from build123d import *

# Parameters (mm, degrees)
EXTRUDE_1_DEPTH     = 2
FILLET_1_R          = 10
SKETCH_3_R          = 2.1
SKETCH_3_R_2        = 5
CUT_EXTRUDE_1_DEPTH = 3


with BuildPart() as part:
    # 草图1 → 凸台-拉伸1 (new body)
    with BuildSketch(Plane.XY):
        Polygon((75, 117), (-75, 117), (-75, 66.5), (-50, 66.5), (-50, 10), (-75, 10), (-75, -117), (75, -117), (75, 10), (50, 10), (50, 66.5), (75, 66.5), align=None)
        with BuildLine():
            Line((-49, -6), (-49, -101))
            ThreePointArc((-49, -101), (-55, -107), (-61, -101))
            Line((-61, -101), (-61, -6))
            ThreePointArc((-61, -6), (-55, 0), (-49, -6))
        make_face(mode=Mode.SUBTRACT)
        with BuildLine():
            Line((49, -6), (49, -101))
            ThreePointArc((49, -101), (55, -107), (61, -101))
            Line((61, -101), (61, -6))
            ThreePointArc((61, -6), (55, 0), (49, -6))
        make_face(mode=Mode.SUBTRACT)
    extrude(amount=EXTRUDE_1_DEPTH)

    # 圆角1
    fillet_1_edges = [part.edges().sort_by_distance(p)[0] for p in [
        (-75, 117, 1),
        (75, 117, 1),
        (75, 66.5, 1),
        (75, 10, 1),
        (75, -117, 1),
        (-75, -117, 1),
        (-75, 10, 1),
        (-75, 66.5, 1),
    ]]
    fillet(fillet_1_edges, radius=FILLET_1_R)

    # 草图3 → 切除-拉伸1 (cut, through all)
    with BuildSketch(Plane.XY.offset(2)):
        with Locations((-10, 102)):
            Circle(SKETCH_3_R)
        with Locations((-35, 38.25)):
            Circle(SKETCH_3_R_2)
        with Locations((-42.425, 30.825757614)):
            Circle(SKETCH_3_R)
        with Locations((-42.424242386, 45.675)):
            Circle(SKETCH_3_R)
        with Locations((-27.575, 45.674242386)):
            Circle(SKETCH_3_R)
        with Locations((-27.575757614, 30.825)):
            Circle(SKETCH_3_R)
        with Locations((27.575757614, 30.825)):
            Circle(SKETCH_3_R)
        with Locations((27.575, 45.674242386)):
            Circle(SKETCH_3_R)
        with Locations((42.424242386, 45.675)):
            Circle(SKETCH_3_R)
        with Locations((42.425, 30.825757614)):
            Circle(SKETCH_3_R)
        with Locations((35, 38.25)):
            Circle(SKETCH_3_R_2)
        with Locations((10, 102)):
            Circle(SKETCH_3_R)
        with Locations((27, -49)):
            Circle(SKETCH_3_R)
        with Locations((-27, -49)):
            Circle(SKETCH_3_R)
        with Locations((-11.5, -102)):
            Circle(SKETCH_3_R)
        with Locations((11.5, -102)):
            Circle(SKETCH_3_R)
        with Locations((11.5, -74)):
            Circle(SKETCH_3_R)
        with Locations((-11.5, -74)):
            Circle(SKETCH_3_R)
        with Locations((-28, 55)):
            Circle(SKETCH_3_R)
        with Locations((28, 55)):
            Circle(SKETCH_3_R)
        with BuildLine():
            Line((-7, 66.5), (7, 66.5))
            ThreePointArc((7, 66.5), (9.121320344, 65.621320344), (10, 63.5))
            Line((10, 63.5), (10, 13))
            ThreePointArc((10, 13), (9.121320344, 10.878679656), (7, 10))
            Line((7, 10), (-7, 10))
            ThreePointArc((-7, 10), (-9.121320344, 10.878679656), (-10, 13))
            Line((-10, 13), (-10, 63.5))
            ThreePointArc((-10, 63.5), (-9.121320344, 65.621320344), (-7, 66.5))
        make_face()
    extrude(amount=-CUT_EXTRUDE_1_DEPTH, mode=Mode.SUBTRACT)


solid = part.part
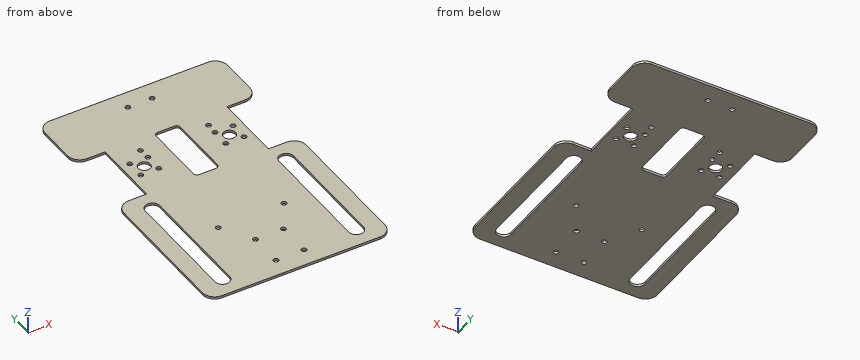
Work out the finished part from the listing and answer in its coordinate system (mm). Coordinates: 2 decimals unless noted, no trailing zeros. Write each loop counter-clockwise with the first axis right and the second up, starting at its lowest first coordinate (ties: lowest second). Pieces come first, ordered by that corner, then holes. Notation, with made-up numbers: M -10,48.25 L 28,48.25 A21 ccw 28,60.25 Z; hole C 63,36.5 d6. An arc over 180 degrees is marked long. Answer as CSV lines item,"result". Start each with the question number.
Item 1: Consider L1, parallel to X at y = -84, z = 1.35; L2, parallel to X at y = 30, z = 0.3; L3, parallel to Y at x = 27, z = 1.6. Determine where each line is inside the solid, lowest interval first.
Item 2: Section A-A on x = -55 is taken. Write down the section's boundary in (y, z).
Item 3: Flat-ended cylindrical pins translate along their axes: P1, Ø6.5, axis at x = -10, y = 102, coming from the +Z side; P2, Ø1, axis at y = 28, z = 1, coming from the -X side. Find the tip coordinate at first contact, or state that the pin passes through.
Item 4: Section D-D on y = 38.25 is taken. Write down the section's boundary in (x, z), and give its area (3 significant figures).
Item 5: Section C-C on x = -35 is taken. Write down the section's boundary in (y, z).
Item 6: Section B-B on y = -11.5 is taken. Write down the section's boundary in (x, z).
Checks:
1,L1,"x = -75 to -61, -49 to 49, 61 to 75"
1,L2,"x = -50 to -44.36, -40.49 to -29.51, -25.64 to -10, 10 to 25.64, 29.51 to 40.49, 44.36 to 50"
1,L3,"y = -117 to -51.1, -46.9 to 28.81, 32.84 to 43.65, 47.69 to 53.15, 56.85 to 117"
2,outline,"M -117,0 L -107,0 L -107,2 L -117,2 Z; M 0,0 L 10,0 L 10,2 L 0,2 Z; M 66.5,0 L 117,0 L 117,2 L 66.5,2 Z"
3,P1,"stops at z = 2"
3,P2,"stops at x = -50"
4,outline,"M -50,0 L -40,0 L -40,2 L -50,2 Z; M -30,0 L -10,0 L -10,2 L -30,2 Z; M 10,0 L 30,0 L 30,2 L 10,2 Z; M 40,0 L 50,0 L 50,2 L 40,2 Z"
4,area,"120 mm²"
5,outline,"M -117,0 L 33.25,0 L 33.25,2 L -117,2 Z; M 43.25,0 L 117,0 L 117,2 L 43.25,2 Z"
6,outline,"M -75,0 L -61,0 L -61,2 L -75,2 Z; M -49,0 L 49,0 L 49,2 L -49,2 Z; M 61,0 L 75,0 L 75,2 L 61,2 Z"
